from build123d import *

# Parameters (mm, degrees)
F0_W     = 85
F0_H     = 55
F1_DEPTH = 5
F2_T     = -2
F3_R     = 1
F4_R     = 1
F5_R     = 1
F6_R     = 1


with BuildPart() as f1:
    # F0 (on Top) → F1 (new body)
    with BuildSketch(Plane.XY):
        Rectangle(F0_W, F0_H)
    extrude(amount=F1_DEPTH)

    # F2
    f2_openings = [f1.faces().sort_by_distance(p)[0] for p in [
        (0, 0, 5),
    ]]
    offset(amount=F2_T, openings=f2_openings)

    # F3
    f3_edges = [f1.edges().sort_by_distance(p)[0] for p in [
        (0, -27.5, 0),
    ]]
    fillet(f3_edges, radius=F3_R)

    # F4
    f4_edges = [f1.edges().sort_by_distance(p)[0] for p in [
        (-42.5, 0.5, 0),
    ]]
    fillet(f4_edges, radius=F4_R)

    # F5
    f5_edges = [f1.edges().sort_by_distance(p)[0] for p in [
        (42.5, 0.5, 0),
    ]]
    fillet(f5_edges, radius=F5_R)

    # F6
    f6_edges = [f1.edges().sort_by_distance(p)[0] for p in [
        (0, 27.5, 0),
    ]]
    fillet(f6_edges, radius=F6_R)


solid = f1.part
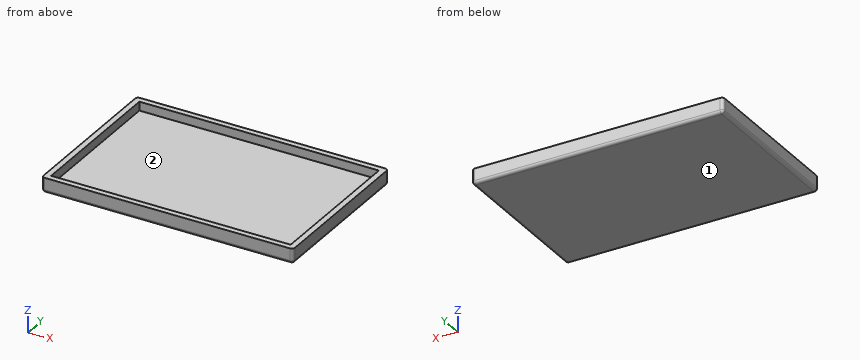
Geometry: final body of the model. Coordinates: model frame, mm. Face numbers are marked on the shaded views. Round coordinates to 2 decimals unless told otherwise and drop trailing zeros. Loops run counter-clockwise (first coordinate to the right, second up) from the corner with the lowest first, then second, coordinate; pieces in that order, holes last. Notation, with made-up numbers: (56.5, 56.25) - (81.5, 56.25) arc R15 ccw to (81.5, 67.25) - close; hole circle Ø10 at (54, -15.5). An arc over 180 degrees is marked (long way). Write each question's results on one line, items separated by ' | '. Start each with the question number.
1) Mould query, pull axis Y, two halves, no side actions, for the marked faces 1 and 2. Classes: released by +Y, released by -Y, zero draft, split by the parting line, or undercut.
2) First-contact query: P1, Ø15.5, axis at x = 10.5, y = 10.5, coming from the +Z side. Flat tip, straight axial feed; report the tip coordinate or a pass-through.
3) Cut plane A-A on y = 18.5. Return loops of the section in (x, z).
4) Cut plane C-C on z = 2.9. Return loops of the section in (x, y), then the cut area to 3 significant figures.
5) Line query: probe 1 along Y at (x, z) = (13, 3.4); probe 2 along X at (y, z) = (-18, 3.55); probe 3 along Z at (x, y) = (34, -3). Output: solid intervals per line, ascending. Write a range as [from, to].
6) Cut plane B-B on x = -9.5. Return loops of the section in (y, z).
Verdict:
1) face 1: zero draft | face 2: undercut
2) P1: stops at z = 2
3) outline: (-42.5, 1) arc R1 ccw to (-41.5, 0) - (41.5, 0) arc R1 ccw to (42.5, 1) - (42.5, 5) - (40.5, 5) - (40.5, 2) - (-40.5, 2) - (-40.5, 5) - (-42.5, 5) - close
4) outline: (-42.5, -26.5) arc R1 ccw to (-41.5, -27.5) - (41.5, -27.5) arc R1 ccw to (42.5, -26.5) - (42.5, 26.5) arc R1 ccw to (41.5, 27.5) - (-41.5, 27.5) arc R1 ccw to (-42.5, 26.5) - close; hole (-40.5, -25.5) - (40.5, -25.5) - (40.5, 25.5) - (-40.5, 25.5) - close | area: 543 mm2
5) probe 1: y = [-27.5, -25.5], [25.5, 27.5] | probe 2: x = [-42.5, -40.5], [40.5, 42.5] | probe 3: z = [0, 2]
6) outline: (-27.5, 1) arc R1 ccw to (-26.5, 0) - (26.5, 0) arc R1 ccw to (27.5, 1) - (27.5, 5) - (25.5, 5) - (25.5, 2) - (-25.5, 2) - (-25.5, 5) - (-27.5, 5) - close
